```python
from build123d import *

# Parameters (mm, degrees)
SCHIZZO1_R                   = 0.936245514
SCHIZZO1_R_2                 = 1
ESTRUSIONE_ESTRUSIONE1_DEPTH = 2.5
RACCORDO1_R                  = 2.7


with BuildPart() as part:
    # Schizzo1 → Estrusione-Estrusione1 (new body)
    with BuildSketch(Plane(origin=(0, 0, 0), x_dir=(1, 0, 0), z_dir=(0, 1, 0))):
        with BuildLine():
            Line((0, 0), (5.035291563, 3.262796174))
            ThreePointArc((5.035291563, 3.262796174), (-4.27091895, 21.690860387), (-21.285586763, 33.382745778))
            Line((-21.285586763, 33.382745778), (-24.592109016, 28.376059189))
            ThreePointArc((-24.592109016, 28.376059189), (-8.523142058, 17.457823812), (0, 0))
        make_face()
        with Locations((-20.099209332, 29.73535462)):
            Circle(SCHIZZO1_R, mode=Mode.SUBTRACT)
        with Locations((1.745777445, 4.706006726)):
            Circle(SCHIZZO1_R_2, mode=Mode.SUBTRACT)
    extrude(amount=ESTRUSIONE_ESTRUSIONE1_DEPTH)

    # Raccordo1
    raccordo1_edges = [part.edges().sort_by_distance(p)[0] for p in [
        (-24.592109016, 1.25, -28.376059189),
        (-21.285586763, 1.25, -33.382745778),
        (5.035291563, 1.25, -3.262796174),
        (0, 1.25, 0),
    ]]
    fillet(raccordo1_edges, radius=RACCORDO1_R)


solid = part.part
```
Verification items for the finished model (mm, model axes). Coordinates: 2 decimals unless noted, no trailing zeros. Loops run counter-clockwise (first coordinate to the right, second up) from the corner with the lowest first, then second, coordinate; pieces in that order, holes last. Notation, with made-up numbers: (64.25, -1.75) - (78.25, -1.75) arc R5 ccw to (78.25, 5.25) - close; hole circle Ø10 at (83, 20.25). An arc over 180 degrees is marked (long way). Put each result on its own line as item: value.
Item 1: Scan lines: line 1 along Z through (x, y) = (2.25, 1.55); line 2 along Z through (x, y) = (-19.25, 1.5); line 3 along X through (y, z) = (1.25, -5.5). Record each from-to range of solid material in increasing order.
Conclusion:
line 1: z = -11.59 to -5.57, -3.84 to -1.68
line 2: z = -32.57 to -30.13, -29.34 to -26.03
line 3: x = -1.52 to 1.14, 2.35 to 4.48
Item 2: Section check B-B (z = -17.5). Enter the section's corners in (x, y).
Conclusion:
outline: (-8.56, 0) - (-1.05, 0) - (-1.05, 2.5) - (-8.56, 2.5) - close
Item 3: Draft check along X on faces 1 (the face through (-20.221, 1.232, -30.664)), 2 (the face through (-20.991, 1.268, -32.657)), 3 (the face through (-8, 2.5, -18)). Enter one of: pulls with the +X half, pulls with the -X half, needs draft (parallel to the pull), parting line crosses it, or undercut.
Conclusion:
face 1: undercut
face 2: parting line crosses it
face 3: needs draft
Item 4: Gauge pin test, flat ends, axial feed: pin 1 Ø1 at (y, z) = (2, -20) entering from +X; pin 2 Ø1 at (y, z) = (1.5, -16.5) entering from +X. Record the tip position at first contact, or that the pin passes through.
Conclusion:
pin 1: stops at x = -2.48
pin 2: stops at x = -0.09
Item 5: Section check A-A (y = 1.3). Enter the section's corners in (x, z), then the cut area to 3 significant figures.
Conclusion:
outline: (-22.77, -31.14) - (-22.5, -31.55) arc R2.7 ccw to (-19.18, -32.54) arc R41.63 ccw to (4.56, -5.19) arc R2.7 ccw to (3.42, -2.22) - (3.18, -2.06) arc R2.7 ccw to (-0.88, -3.55) arc R37.8 cw to (-21.62, -27.19) arc R2.7 ccw to start; hole circle Ø1.87 at (-20.1, -29.74); hole circle Ø2 at (1.75, -4.71)
area: 226 mm2
Item 6: Section check C-C (x = -8.5). Enter the section's corners in (y, z), then the cut area to 3 significant figures.
Conclusion:
outline: (0, -25.88) - (2.5, -25.88) - (2.5, -17.43) - (0, -17.43) - close
area: 21.1 mm2
